```python
from build123d import *

# Parameters (mm, degrees)
SKETCH1_R      = 2.35
EXTRUDE1_DEPTH = 3.1


with BuildPart() as part:
    # Sketch1 → Extrude1 (new body)
    with BuildSketch(Plane.XY):
        with BuildLine():
            Line((-37.138157114, 29.933489293), (-14.388157114, 29.933489293))
            ThreePointArc((-14.388157114, 29.933489293), (-10.78087227, 27.473805885), (-11.7530861, 23.217358224))
            Line((-11.7530861, 23.217358224), (-23.1280861, 12.667358224))
            ThreePointArc((-23.1280861, 12.667358224), (-25.763157114, 11.633489293), (-28.398228128, 12.667358224))
            Line((-28.398228128, 12.667358224), (-39.773228128, 23.217358224))
            ThreePointArc((-39.773228128, 23.217358224), (-40.745441958, 27.473805885), (-37.138157114, 29.933489293))
        make_face()
        with Locations(Location((-14.388157114, 26.058489293, 0), (0, 0, 180))):
            Circle(SKETCH1_R, mode=Mode.SUBTRACT)
        with Locations(Location((-37.138157114, 26.058489293, 0), (0, 0, 180))):
            Circle(SKETCH1_R, mode=Mode.SUBTRACT)
        with Locations(Location((-25.763157114, 15.508489293, 0), (0, 0, 180))):
            Circle(SKETCH1_R, mode=Mode.SUBTRACT)
        with BuildLine():
            Line((-33.76750302, 22.568552775), (-29.341459115, 18.664654654))
            ThreePointArc((-29.341459115, 18.664654654), (-28.720659193, 18.415441082), (-28.081652728, 18.613356938))
            ThreePointArc((-28.081652728, 18.613356938), (-25.763157114, 19.383489293), (-23.4446615, 18.613356938))
            ThreePointArc((-23.4446615, 18.613356938), (-22.805655035, 18.415441082), (-22.184855112, 18.664654654))
            Line((-22.184855112, 18.664654654), (-17.758811208, 22.568552775))
            ThreePointArc((-17.758811208, 22.568552775), (-17.428169762, 23.19327051), (-17.593190704, 23.880558008))
            ThreePointArc((-17.593190704, 23.880558008), (-17.954657824, 24.543333299), (-18.180755673, 25.263617499))
            ThreePointArc((-18.180755673, 25.263617499), (-18.529065613, 25.834739319), (-19.159490785, 26.058489293))
            Line((-19.159490785, 26.058489293), (-32.366823443, 26.058489293))
            ThreePointArc((-32.366823443, 26.058489293), (-32.997248615, 25.834739319), (-33.345558555, 25.263617499))
            ThreePointArc((-33.345558555, 25.263617499), (-33.571656404, 24.543333299), (-33.933123524, 23.880558008))
            ThreePointArc((-33.933123524, 23.880558008), (-34.098144466, 23.19327051), (-33.76750302, 22.568552775))
        make_face(mode=Mode.SUBTRACT)
    extrude(amount=EXTRUDE1_DEPTH)


solid = part.part
```
Build history of the part. All positions in model axes, mm. A direction names the side the tool comes from. Round coordinates to 2 decimals unless told otherwise and drop trailing zeros. Write each loop counter-clockwise with the first axis right and the second up, starting at its lowest first coordinate (ties: lowest second). Pieces come first, ordered by that corner, then holes.
1) Drill centre lines: probe 1 along X at (y, z) = (19, 2.4); probe 2 along Y at (x, z) = (-26, 1.6); probe 3 along X at (y, z) = (18.75, 1.55). Where is each one in solid material? Low to high.
2) Mould opens along X. For faces 3 (the cylindrical face through (-25.723, 11.634, 1.528)), 4 (the cylindrical face through (-14.08, 23.73, 1.53)), 5 (the flat face through (-17.361, 18.016, 1.528)), 6 (the flat face through (-26, 27, 3.1)) say: +X half, -X half, draft (parallel to the pull), parting line (faces both ways), or undercut.
3) Band-saw the part on B-B, the plane y = 26.5. List the corners of the cut face in (x, z).
4) Band-saw the part on A-A, the plane x = -25. List the corners of the cut face in (y, z).
5) 3-axis set-ups, long thin cutter, end or side, ignore diameter. For faces 1 (the cylindrical face through (-40.77, 27.41, 1.53)), 2 (the cylindrical face through (-33.57, 24.55, 1.53)): which of +Z, -Z, +X, -X, +Y, -Y reach the whole face in a straight line?
6) Band-saw the part on D-D, the plane x = -29. List the corners of the cut face in (y, z), and give its area (3 significant figures).
7) Pin check, flat tips, straight feed: pin 1 (1 mm diameter, centred on y = 16.5, z = 2, fed in from +X); pin 2 (7.5 mm diameter, centred on x = -37.14, y = 26.06, fed in from -Z); pin 3 (4 mm diameter, centred on x = -25.76, y = 15.51, fed in from -Z). Stop position of each tip, or through.
8) Band-saw the part on C-C, the plane y = 24.5. List the corners of the cut face in (x, z).
Ans:
1. probe 1: x = -35.23 to -29.72, -27.44 to -24.08, -21.8 to -16.3
1. probe 2: y = 11.64 to 13.17, 17.85 to 19.38, 26.06 to 29.93
1. probe 3: x = -34.96 to -29.44, -27.89 to -23.64, -22.09 to -16.57
2. face 3: parting line
2. face 4: undercut
2. face 5: +X half
2. face 6: draft
3. outline: (-40.99, 0) - (-39.45, 0) - (-39.45, 3.1) - (-40.99, 3.1) - close; (-34.83, 0) - (-16.7, 0) - (-16.7, 3.1) - (-34.83, 3.1) - close; (-12.08, 0) - (-10.54, 0) - (-10.54, 3.1) - (-12.08, 3.1) - close
4. outline: (11.71, 0) - (13.29, 0) - (13.29, 3.1) - (11.71, 3.1) - close; (17.73, 0) - (19.31, 0) - (19.31, 3.1) - (17.73, 3.1) - close; (26.06, 0) - (29.93, 0) - (29.93, 3.1) - (26.06, 3.1) - close
5. face 1: +Z, -Z, -X
5. face 2: +Z, -Z
6. outline: (13.23, 0) - (18.47, 0) - (18.47, 3.1) - (13.23, 3.1) - close; (26.06, 0) - (29.93, 0) - (29.93, 3.1) - (26.06, 3.1) - close
6. area: 28.3 mm2
7. pin 1: stops at x = -18.46
7. pin 2: stops at z = 0
7. pin 3: passes through
8. outline: (-40.69, 0) - (-38.9, 0) - (-38.9, 3.1) - (-40.69, 3.1) - close; (-35.38, 0) - (-33.59, 0) - (-33.59, 3.1) - (-35.38, 3.1) - close; (-17.94, 0) - (-16.15, 0) - (-16.15, 3.1) - (-17.94, 3.1) - close; (-12.63, 0) - (-10.84, 0) - (-10.84, 3.1) - (-12.63, 3.1) - close
